Verification items for the finished model (mm, model axes). A direction names the side the tool comes from. Coordinates: 2 decimals unless noted, no trailing zeros. Order: outer loops, then holes, each group sorted by start corner. A loop starts at its lowest first (then second) coordinate and runs counter-clockwise, first axis right, second up. Notation, with made-up numbers: (42, -16) -> (92, -16) arc R12 ccw to (92, -11) -> close; hole circle Ø5 at (-16, -29). An arc over 180 degrees is marked (long way). Write item = value, one per line. Start each with the question number.
from build123d import *

# Parameters (mm, degrees)
SKETCH_2_R          = 6
CUT_EXTRUDE_1_DEPTH = 4
SKETCH_3_R          = 3.1
CUT_EXTRUDE_2_DEPTH = 16.779733838


with BuildPart() as part:
    # 草图1 → 旋转1 (revolve)
    with BuildSketch(Plane(origin=(0, 0, 0), x_dir=(1, 0, 0), z_dir=(0, 1, 0)), mode=Mode.PRIVATE) as revolve_1_sk:
        Polygon((-7.5, 9), (-5, 6.5), (-7.5, 4), (-10, 1.5), (-10, 0), (0, 0), (0, 11), (-7.5, 11), align=None)
    revolve(revolve_1_sk.sketch.rotate(Axis((0, 0, 1000), (0, 0, -1)), 180), axis=Axis((0, 0, 1000), (0, 0, -1)))

    # 草图2 → 切除-拉伸1 (cut)
    with BuildSketch(Plane.XY):
        Circle(SKETCH_2_R)
    extrude(amount=-CUT_EXTRUDE_1_DEPTH, mode=Mode.SUBTRACT)

    # 草图3 → 切除-拉伸2 (cut, through all)
    with BuildSketch(Plane.XY.offset(-4)):
        Circle(SKETCH_3_R)
    extrude(amount=-CUT_EXTRUDE_2_DEPTH, mode=Mode.SUBTRACT)


solid = part.part
Item 1: Gauge pin test, flat ends, axial feed: P1, Ø10, axis at x = -1.5, y = -4, coming from the +Z side; P2, Ø9.5, axis at x = -0.5, y = 1, coming from the +Z side; P3, Ø3.5, axis at x = 0, y = 0, coming from the -Z side; P4, Ø5, axis at x = -7.5, z = -5, coming from the +Y side. Record the tip position at first contact, or that the pin passes through.
Item 2: Section check C-C (z = -5.5). Record the boundary of the cut face in (x, y), then the cut area to 3 significant figures.
Item 3: Mould release check, pull along Z, two halves, no side actions. Record for faces 1 (the cylindrical face through (1.43, -2.75, -7.45)), 2 (the conical face through (2.363, 4.544, -6.621)), 3 (the flat face through (7, 0, 0)): pulls with the +Z half, pulls with the -Z half, needs draft (parallel to the pull), parting line crosses it, or undercut.
Item 4: Section check A-A (x = 0). Record the boundary of the cut face in (y, z).
Item 5: Tool access check on faces 4 (the cylindrical face through (-6, 0, -2)), 5 (the cylindrical face through (-10, 0, -1)), 6 (the cylindrical face through (4.032, -6.324, -9.986)), 7 (the conical face through (-4.216, 3.233, -6.187)). Record the directions out of +Z, -Z, +X, -X, +Y, -Y that give a thin tool (end or side, any length) a straight path to the whole face; none if there is none.
Item 6: Thickness scan on line 1 (Z direction, x = -3.5, y = -3); line 2 (Y direction, x = 1.25, z = -6); line 3 (Z direction, x = 1.5, y = -7). Record the ranges inside material, lowest first.
Item 7: Section check D-D (z = -4.25). Record the boundary of the cut face in (x, y), then the cut area to 3 significant figures.
Filled sheet:
q1.P1 = 0
q1.P2 = -4
q1.P3 = through
q1.P4 = 6.02
q2.outline = circle Ø12 at (0, 0); hole circle Ø6.2 at (0, 0)
q2.area = 82.9 mm^2
q3.face_1 = needs draft
q3.face_2 = undercut
q3.face_3 = pulls with the +Z half
q4.outline = (-10, -1.5) -> (-5, -6.5) -> (-7.5, -9) -> (-7.5, -11) -> (-3.1, -11) -> (-3.1, -4) -> (-6, -4) -> (-6, 0) -> (-10, 0) -> close; (3.1, -11) -> (7.5, -11) -> (7.5, -9) -> (5, -6.5) -> (10, -1.5) -> (10, 0) -> (6, 0) -> (6, -4) -> (3.1, -4) -> close
q5.face_4 = +Z
q5.face_5 = +Z, -Z
q5.face_6 = -Z
q5.face_7 = none
q6.line_1 = -11 to -4
q6.line_2 = -5.36 to -2.84, 2.84 to 5.36
q6.line_3 = -11 to -8.66, -4.34 to 0
q7.outline = circle Ø14.5 at (0, 0); hole circle Ø6.2 at (0, 0)
q7.area = 135 mm^2
